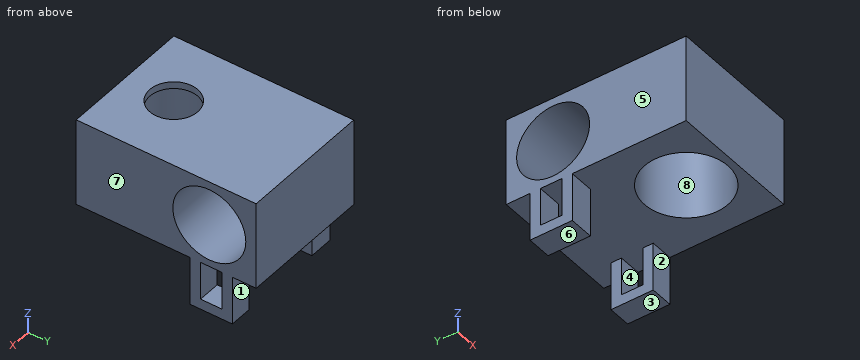
```python
from build123d import *

# Parameters (mm, degrees)
F0_W     = 25.8862247349
F0_H     = 12.6448004093
F0_R     = 5.25
F1_DEPTH = 19.05
F3_DEPTH = 1
F4_START = -1
F4_DEPTH = 24.4
F6_DEPTH = 3.2512
F7_START = -15.5194
F7_DEPTH = 3.5306


with BuildPart() as f1:
    # F0 (on Right) → F1 (new body)
    with BuildSketch(Plane.YZ):
        with Locations((-3.152461024, -0.6018574079)):
            Rectangle(F0_W, F0_H)
        with Locations((3.0532879755, -0.688746688)):
            Circle(F0_R, mode=Mode.SUBTRACT)
    extrude(amount=F1_DEPTH)

    # F2 (on face) → F3 (cut)
    with BuildSketch(Plane.XY.offset(5.7205427967)):
        with BuildLine():
            Line((9.525, -9.0865883976), (12.975, -9.0865883976))
            ThreePointArc((12.975, -9.0865883976), (9.525, -5.6365883976), (6.075, -9.0865883976))
            Line((6.075, -9.0865883976), (9.525, -9.0865883976))
        make_face()
        with BuildLine():
            ThreePointArc((6.075, -9.0865883976), (9.525, -12.5365883976), (12.975, -9.0865883976))
            Line((12.975, -9.0865883976), (9.525, -9.0865883976))
            Line((9.525, -9.0865883976), (6.075, -9.0865883976))
        make_face()
    extrude(amount=-F3_DEPTH, mode=Mode.SUBTRACT)

    # F2 (on face) → F4 (cut)
    with BuildSketch(Plane.XY.offset(5.7205427967).offset(F4_START)):
        with BuildLine():
            Line((15.525, -9.0865883976), (12.975, -9.0865883976))
            ThreePointArc((12.975, -9.0865883976), (9.525, -12.5365883976), (6.075, -9.0865883976))
            Line((6.075, -9.0865883976), (3.525, -9.0865883976))
            ThreePointArc((3.525, -9.0865883976), (9.525, -15.0865883976), (15.525, -9.0865883976))
        make_face()
        with BuildLine():
            Line((9.525, -9.0865883976), (12.975, -9.0865883976))
            ThreePointArc((12.975, -9.0865883976), (9.525, -5.6365883976), (6.075, -9.0865883976))
            Line((6.075, -9.0865883976), (9.525, -9.0865883976))
        make_face()
        with BuildLine():
            ThreePointArc((6.075, -9.0865883976), (9.525, -5.6365883976), (12.975, -9.0865883976))
            Line((12.975, -9.0865883976), (15.525, -9.0865883976))
            ThreePointArc((15.525, -9.0865883976), (9.525, -3.0865883976), (3.525, -9.0865883976))
            Line((3.525, -9.0865883976), (6.075, -9.0865883976))
        make_face()
        with BuildLine():
            ThreePointArc((6.075, -9.0865883976), (9.525, -12.5365883976), (12.975, -9.0865883976))
            Line((12.975, -9.0865883976), (9.525, -9.0865883976))
            Line((9.525, -9.0865883976), (6.075, -9.0865883976))
        make_face()
    extrude(amount=-F4_DEPTH, mode=Mode.SUBTRACT)

    # F5 (on face) → F6 (join)
    with BuildSketch(Plane.YZ.offset(19.05)):
        Polygon((6.3707139343, -13.9242576137), (6.3707139343, -6.9242576137), (4.8707139343, -6.9242576126), (4.8707139343, -12.4242576137), (1.7881980821, -12.4242576137), (1.7881980821, -6.9242576137), (0.2881980821, -6.9242576126), (0.2881980821, -13.9242576137), align=None)
    extrude(amount=-F6_DEPTH)

    # F5 (on face) → F7 (join)
    with BuildSketch(Plane.YZ.offset(19.05).offset(F7_START)):
        Polygon((6.3707139343, -13.9242576137), (6.3707139343, -6.9242576137), (4.8707139343, -6.9242576126), (4.8707139343, -12.4242576137), (1.7881980821, -12.4242576137), (1.7881980821, -6.9242576137), (0.2881980821, -6.9242576126), (0.2881980821, -13.9242576137), align=None)
    extrude(amount=-F7_DEPTH)


solid = f1.part
```
Geometry check sheet. Reference: the model listing, model coordinates, mm. Face numbers are marked on the shaded views. A direction names the side the tool comes from. Round coordinates to 2 decimals unless told otherwise and drop trailing zeros. Order: outer loops, then holes, each group sorted by start corner. A loop starts at its lowest first (then second) coordinate and runs counter-clockwise, first axis right, second up. Notation, with made-up numbers: (67.5, -10.75) - (84.5, -10.75) arc R10 cw to (84.5, -1.75) - close; hole circle Ø4 at (-37, 19.25). An arc over 180 degrees is marked (long way). Use a Markdown table: item, result. Add a question column.
(1) Tool access check on the marked faces 1, 2, 3 and 4. Record the directions out of +Z, -Z, +X, -X, +Y, -Y that give a thin tool (end or side, any length) a straight path to the whole face; none if there is none.
(2) Sectioned sample at A-A, the plane z = -7.5. Enter the section's corners in (x, y).
(3) Sectioned sample at B-B, the plane x = 10.25. Enter the section's corners in (y, z).
(4) Sectioned sample at D-D, the plane y = -8.75. Enter the section's corners in (x, z).
(5) Sectioned sample at C-C, the plane z = 2.25. Enter the section's corners in (x, y) (3 decimals).
(6) Material ranges on line 1 along Y through (x, z) = (4.25, -5.25); line 2 along Y through (x, z) = (9.5, -3.5); line 3 along Y through (x, z) = (1.25, -10.75), recorded low to high. Write a range as [from, to].
(7) Depth check by flat-ended pin: pin 1 (1 mm diameter, centred on x = 17.5, z = -9.5, fed in from -Y); pin 2 (2.5 mm diameter, centred on x = 16.5, z = -9.5, fed in from +Y); pin 3 (9.5 mm diameter, centred on x = 7.5, y = -9.5, fed in from -Z); pin 4 (1.5 mm diameter, centred on y = -4.5, z = -2, fed in from -X). Enter the tip coordinate at first touch or a pass-through.
(8) Release check for a two-part mould opening along X. For the marked faces 5, 6, 7 and 8 record: pulls with the +X half, pulls with the -X half, needs draft (parallel to the pull), parting line crosses it, or undercut.
Answers below:
| question | item | result |
|---|---|---|
| 1 | face 1 | -Z, +X, -X, +Y |
| 1 | face 2 | -Z, +X, -X, -Y |
| 1 | face 3 | -Z, +X, -X, +Y, -Y |
| 1 | face 4 | +X, -X |
| 2 | outline | (0, 0.29) - (3.53, 0.29) - (3.53, 1.79) - (0, 1.79) - close; (0, 4.87) - (3.53, 4.87) - (3.53, 6.37) - (0, 6.37) - close; (15.8, 0.29) - (19.05, 0.29) - (19.05, 1.79) - (15.8, 1.79) - close; (15.8, 4.87) - (19.05, 4.87) - (19.05, 6.37) - (15.8, 6.37) - close |
| 3 | outline | (-16.1, -6.92) - (-15.04, -6.92) - (-15.04, 4.72) - (-12.46, 4.72) - (-12.46, 5.72) - (-16.1, 5.72) - close; (-5.71, 4.72) - (-3.13, 4.72) - (-3.13, -6.92) - (9.79, -6.92) - (9.79, 5.72) - (-5.71, 5.72) - close; hole circle Ø10.5 at (3.05, -0.69) |
| 4 | outline | (0, -6.92) - (3.53, -6.92) - (3.53, 4.72) - (6.09, 4.72) - (6.09, 5.72) - (0, 5.72) - close; (12.96, 4.72) - (15.52, 4.72) - (15.52, -6.92) - (19.05, -6.92) - (19.05, 5.72) - (12.96, 5.72) - close |
| 5 | outline | (0, -16.096) - (19.05, -16.096) - (19.05, -1.297) - (0, -1.297) - close; (0, 7.404) - (19.05, 7.404) - (19.05, 9.791) - (0, 9.791) - close; hole circle Ø12 at (9.525, -9.087) |
| 6 | line 1 | [-16.1, -11.95], [-6.23, 0.45], [5.65, 9.79] |
| 6 | line 2 | [-16.1, -15.09], [-3.09, -1.38], [7.49, 9.79] |
| 6 | line 3 | [0.29, 1.79], [4.87, 6.37] |
| 7 | pin 1 | y = 0.29 |
| 7 | pin 2 | y = 6.37 |
| 7 | pin 3 | z = -6.92 |
| 7 | pin 4 | x = 0 |
| 8 | face 5 | pulls with the -X half |
| 8 | face 6 | needs draft |
| 8 | face 7 | pulls with the +X half |
| 8 | face 8 | undercut |
